Source: CAD feature listing. Evaluate the final solid. Frame: model axes, mm. Give positions to 0.01 mm unless a question says otherwise; leave off trailing zeros. Order: outer loops, then holes, each group sorted by start corner. A loop starts at its lowest first (then second) coordinate and runs counter-clockwise, first axis right, second up. Notation, with made-up numbers: (87.25, 83) -> (121.25, 83) arc R25 cw to (121.25, 117) -> close; hole circle Ø10 at (16, -1.5). An arc over 180 degrees is marked (long way). Use CSV: the item, a comma, the result in double quotes.
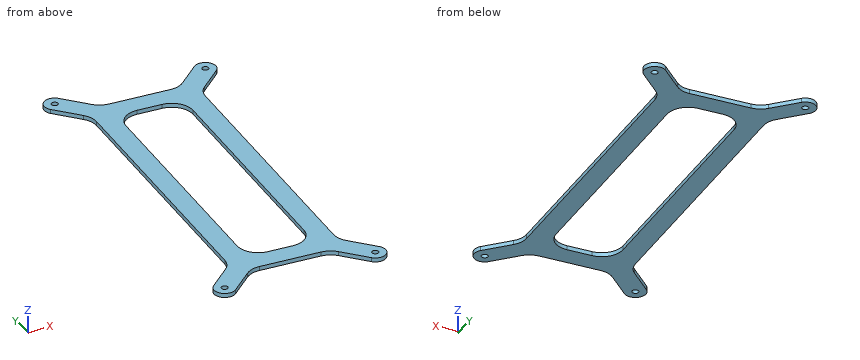
```python
from build123d import *

# Parameters (mm, degrees)
SKETCH1_R           = 1.55
BOSS_EXTRUDE1_DEPTH = 2


with BuildPart() as part:
    # Sketch1 → Boss-Extrude1 (new body)
    with BuildSketch(Plane.XY):
        with BuildLine():
            ThreePointArc((25.385066163, -73.812983116), (23.373646331, -70.469589068), (22.794798226, -66.610958693))
            Line((22.794798226, -66.610958693), (29.003615503, 64.151484254))
            ThreePointArc((29.003615503, 64.151484254), (29.945463503, 67.93790946), (32.264619787, 71.075680584))
            Line((32.264619787, 71.075680584), (43.399330006, 81.200932599))
            ThreePointArc((43.399330006, 81.200932599), (43.738051861, 88.334674079), (36.604310381, 88.673395935))
            Line((36.604310381, 88.673395935), (25.469600163, 78.54814392))
            ThreePointArc((25.469600163, 78.54814392), (22.126206115, 76.536724088), (18.267575741, 75.957875984))
            Line((18.267575741, 75.957875984), (-10.988406497, 77.346998456))
            ThreePointArc((-10.988406497, 77.346998456), (-14.774831703, 78.288846456), (-17.912602827, 80.60800274))
            Line((-17.912602827, 80.60800274), (-28.037854841, 91.742712958))
            ThreePointArc((-28.037854841, 91.742712958), (-35.171596321, 92.081434814), (-35.510318177, 84.947693334))
            Line((-35.510318177, 84.947693334), (-25.385066163, 73.812983116))
            ThreePointArc((-25.385066163, 73.812983116), (-23.373646331, 70.469589068), (-22.794798226, 66.610958693))
            Line((-22.794798226, 66.610958693), (-29.003615503, -64.151484254))
            ThreePointArc((-29.003615503, -64.151484254), (-29.945463503, -67.93790946), (-32.264619787, -71.075680584))
            Line((-32.264619787, -71.075680584), (-43.399330005, -81.200932599))
            ThreePointArc((-43.399330005, -81.200932599), (-43.738051861, -88.334674079), (-36.604310381, -88.673395935))
            Line((-36.604310381, -88.673395935), (-25.469600163, -78.54814392))
            ThreePointArc((-25.469600163, -78.54814392), (-22.126206115, -76.536724088), (-18.26757574, -75.957875984))
            Line((-18.26757574, -75.957875984), (10.988406497, -77.346998456))
            ThreePointArc((10.988406497, -77.346998456), (14.774831703, -78.288846456), (17.912602827, -80.60800274))
            Line((17.912602827, -80.60800274), (28.037854841, -91.742712958))
            ThreePointArc((28.037854841, -91.742712958), (35.171596321, -92.081434814), (35.510318177, -84.947693334))
            Line((35.510318177, -84.947693334), (25.385066163, -73.812983116))
        make_face()
        with BuildLine():
            ThreePointArc((-9.087016293, -66.382517954), (-16.011212623, -63.121513669), (-18.601480559, -55.919489247))
            Line((-18.601480559, -55.919489247), (-13.219440196, 57.430399246))
            ThreePointArc((-13.219440196, 57.430399246), (-9.958435912, 64.354595576), (-2.756411489, 66.944863512))
            Line((-2.756411489, 66.944863512), (9.087016293, 66.382517954))
            ThreePointArc((9.087016293, 66.382517954), (16.011212623, 63.121513669), (18.601480559, 55.919489247))
            Line((18.601480559, 55.919489247), (13.219440196, -57.430399246))
            ThreePointArc((13.219440196, -57.430399246), (9.958435912, -64.354595576), (2.756411489, -66.944863512))
            Line((2.756411489, -66.944863512), (-9.087016293, -66.382517954))
        make_face(mode=Mode.SUBTRACT)
        with Locations((31.774086509, -88.345203146)):
            Circle(SKETCH1_R, mode=Mode.SUBTRACT)
        with Locations((-40.001820193, -84.937164267)):
            Circle(SKETCH1_R, mode=Mode.SUBTRACT)
        with Locations((40.001820193, 84.937164267)):
            Circle(SKETCH1_R, mode=Mode.SUBTRACT)
        with Locations((-31.774086509, 88.345203146)):
            Circle(SKETCH1_R, mode=Mode.SUBTRACT)
    extrude(amount=BOSS_EXTRUDE1_DEPTH)


solid = part.part
```
1. Section query A-A on y = 41. Return loops of the section in (x, z), plus the area to 3 significant figures.
Answer below:
outline,"(-24.01, 0) -> (-14, 0) -> (-14, 2) -> (-24.01, 2) -> close; (17.89, 0) -> (27.9, 0) -> (27.9, 2) -> (17.89, 2) -> close"
area,"40.0 mm²"
2. Section query C-C on z = 1.55. Count the separate pieces of the cut face and the enclosed holes in it, plus the area to 3 significant figures.
Answer below:
separate pieces,"1"
enclosed holes,"5"
area,"4,610 mm²"
3. Pin query (flat end, axial travel): P1, Ø1, axis at y = 0.5, z = 1.5, coming from the -X side. Return the tip coordinate at first contact, or that it passes through.
Answer below:
P1,"stops at x = -25.96"
4. Ray query, line 1 along Y through (x, z) = (33, 1.75); line 2 along Y through (x, z) = (12.5, 1.2); line 3 along Y through (x, z) = (-9, 0.45). Return the intervals inside material, ascending.
Answer below:
line 1,"y = -93.24 to -89.29, -87.4 to -82.19, 71.74 to 85.4"
line 2,"y = -77.53 to -60.71, 65.61 to 76.23"
line 3,"y = -76.4 to -66.39, 65.12 to 77.25"
5. Section query B-B on x = -16. Return loops of the section in (y, z).
Answer below:
outline,"(-76.07, 0) -> (-63.13, 0) -> (-63.13, 2) -> (-76.07, 2) -> close; (-1.13, 0) -> (78.97, 0) -> (78.97, 2) -> (-1.13, 2) -> close"
